Geometry: final body of the model. Coordinates: model frame, mm. A direction names the side the tool comes from. Round coordinates to 2 decimals unless told otherwise and drop trailing zeros. Order: outer loops, then holes, each group sorted by start corner. A loop starts at its lowest first (then second) coordinate and runs counter-clockwise, first axis right, second up. Notation, with made-up numbers: M 32,-7.75 L 61,-7.75 A13 ccw 61,0.25 Z; hole C 83,-1 d6. An arc over 180 degrees is marked long. Put each result on its own line as item: value. Start each with the question number.
1) Material intervals for probe 1 along X at (y, z) = (86, 0); probe 2 along Y at (x, z) = (5, -16.5), sorted ascending. Write a range as [from, to].
2) First-contact query: P1, Ø11.5, axis at x = -5.5, z = -3.5, coming from the +Y side. Flat tip, straight axial feed; report the tip coordinate or a pass-through.
3) Access query for faces 5 (the flat face through (16, 101.6, -18)), 6 (the cylindrical face through (15.12, 91.37, 11.59)). Directions: +Z, -Z, +X, -X, +Y, -Y. A direction counts if a zero-diameter tool reaches every point of the face in a straight line with its end or side. Return the directions, or none.
4) Section A-A, the plane y = 86.5. Return loops of the section in (x, z), then the cut area to 3 significant figures.
5) Draft query along X for faces 1 (the flat face through (76.2, 50, 1)), 2 (the flat face through (-1, 0, -1)), 3 (the flat face through (0, 25.4, 0)), 4 (the flat face through (-76.2, 50, 1)). Return one class per face: pulls with the +X half, pulls with the -X half, needs draft (parallel to the pull), parting line crosses it, or undercut.
from build123d import *

# Parameters (mm, degrees)
SKETCH1_W           = 152.4
SKETCH1_H           = 152.4
BOSS_EXTRUDE1_DEPTH = 101.6


with BuildPart() as part:
    # Sketch1 → Boss-Extrude1 (new body)
    with BuildSketch(Plane(origin=(0, 0, 0), x_dir=(1, 0, 0), z_dir=(0, 1, 0))):
        Rectangle(SKETCH1_W, SKETCH1_H)
    extrude(amount=BOSS_EXTRUDE1_DEPTH)

    # Sketch3 → Cut-Revolve4 (revolve, cut)
    with BuildSketch(Plane.XY):
        with BuildLine():
            Line((-19.05, 80.853685298), (-19.05, 101.6))
            Line((-19.05, 101.6), (0, 101.6))
            Line((0, 101.6), (0, 25.4))
            Line((0, 25.4), (-19.05, 25.4))
            ThreePointArc((-19.05, 25.4), (-44.361028612, 48.675892989), (-23.283333333, 75.844737748))
            ThreePointArc((-23.283333333, 75.844737748), (-20.250085912, 77.574559398), (-19.05, 80.853685298))
        make_face()
    revolve(axis=Axis((0, 101.6, 0), (0, -1, 0)), mode=Mode.SUBTRACT)


solid = part.part
Result sheet:
1. probe 1: x = [-76.2, -19.05], [19.05, 76.2]
1. probe 2: y = [0, 25.4]
2. P1: stops at y = 25.4
3. face 5: +Z, -Z, +X, -X, +Y
3. face 6: +Y
4. outline: M -76.2,-76.2 L 76.2,-76.2 L 76.2,76.2 L -76.2,76.2 Z; hole C 0,0 d38.1
4. area: 22,100 mm2
5. face 1: pulls with the +X half
5. face 2: needs draft
5. face 3: undercut
5. face 4: pulls with the -X half
